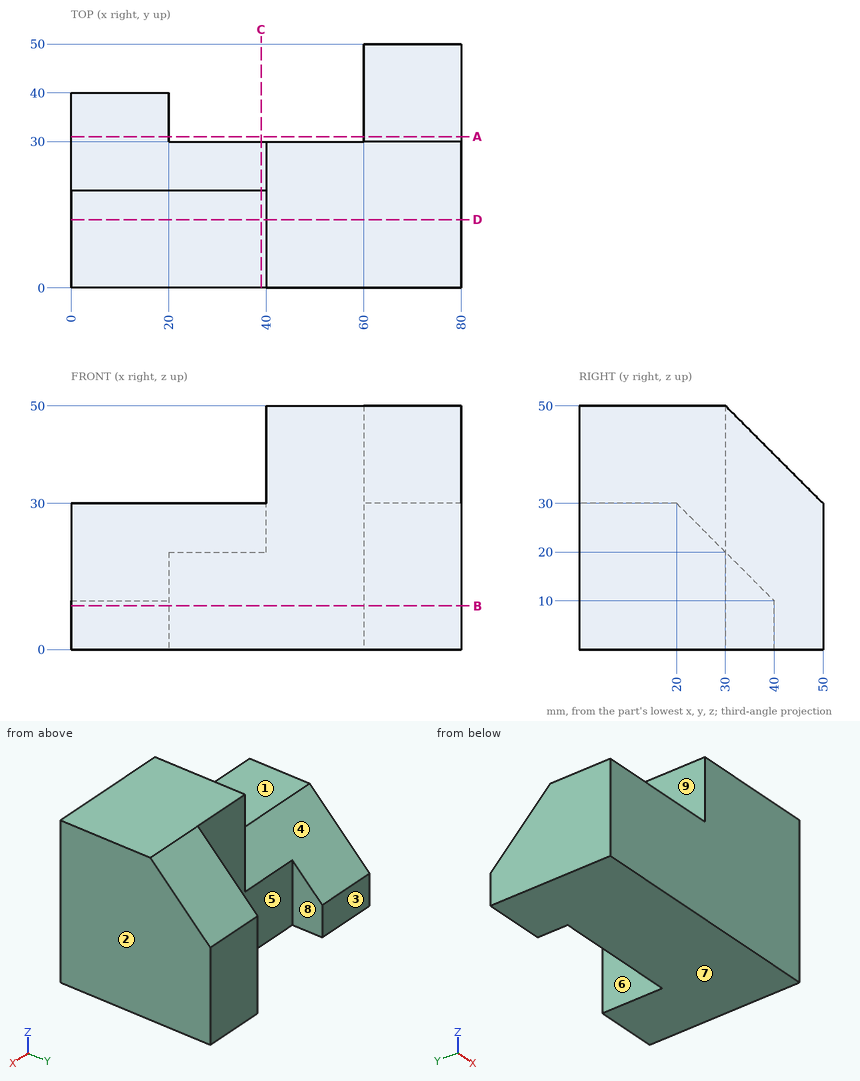
Could you check a few things on this drawing? It's one solid part, dimensions in mm from its lowest x, y, z. A direction names the side the tool comes from. Round coordinates to 2 decimals unless told otherwise and drop trailing zeros. Loops run counter-clockwise (first coordinate to the right, second up) from the corner with the lowest first, then second, coordinate; pieces in that order, holes last. Notation, with made-up numbers: M 67.25,32.5 L 108.25,32.5 A19 cw 108.25,45.5 Z; hole C -26.5,-39 d8. An arc over 180 degrees is marked long. Write each question's results on one line, items separated by ' | '. Start each with the question number.
(1) If I drill on probe 1 along Y at (x, z) = (49, 24.5); probe 2 along X at (y, z) = (39.5, 12); probe 3 along X at (y, z) = (16.5, 45), over which ranges is the centre line in solid material (lowest first)? Write a range as from..to.
(2) On a 3-axis mill with a long thin cutter (end or side, diameter ignored), from which of +Z, -Z, +X, -X, +Y, -Y can I reach the whole of each face in a straight line? I mean the marked faces 1, 2, 3, 4 and 5. Say none if no direction works.
(3) I want a section at B-B (z = 9). Please give me the cut outline in (x, y), then the cut area to 3 significant figures.
(4) I want a section at A-A (y = 31). Please give me the cut outline in (x, z).
(5) Thinking about a two-plate mould opening in X: for the marked faces 6, 7, 8 and 9, which applies, pulls with the +X half, pulls with the -X half, needs draft (parallel to the pull), parting line crosses it, or undercut?
(6) I want a section at C-C (x = 39). Please give me the cut outline in (y, z), then the cut area to 3 significant figures.
(7) Will these pins go through, and if not, where does the flat tip stop? P1, Ø10, axis at x = 16, y = 5, coming from the +Z side; P2, Ø11, axis at x = 10.5, z = 7, coming from the +Y side; P3, Ø6, axis at x = 17, z = 14, coming from the +Y side.
(8) I want a section at D-D (y = 14). Please give me the cut outline in (x, z), then the cut area to 3 significant figures.
Solved:
1) probe 1: y = 0..30 | probe 2: x = 60..80 | probe 3: x = 40..80
2) face 1: +Z, -X, +Y, -Y | face 2: +Z, -Z, +X, +Y, -Y | face 3: +Z, -Z, -X, +Y | face 4: +Z, -X, +Y | face 5: +Z, -Z, +Y
3) outline: M 0,0 L 80,0 L 80,50 L 60,50 L 60,30 L 20,30 L 20,40 L 0,40 Z | area: 3,000 mm²
4) outline: M 0,0 L 20,0 L 20,19 L 0,19 Z; M 60,0 L 80,0 L 80,49 L 60,49 Z
5) face 6: undercut | face 7: needs draft | face 8: undercut | face 9: pulls with the -X half
6) outline: M 0,0 L 30,0 L 30,20 L 20,30 L 0,30 Z | area: 850 mm²
7) P1: stops at z = 30 | P2: stops at y = 40 | P3: stops at y = 39
8) outline: M 0,0 L 80,0 L 80,50 L 40,50 L 40,30 L 0,30 Z | area: 3,200 mm²
